The drawing under review shows one solid part. Ordinate dimensions are in mm from its lowest x, y, z. A direction names the side the tool comes from. Round coordinates to 2 decimals unless told otherwise and drop trailing zeros. Order: outer loops, then holes, each group sorted by start corner. A loop starts at its lowest first (then second) coordinate and runs counter-clockwise, first axis right, second up. Notation, with made-up numbers: M 78.5,35.25 L 123.5,35.25 A22 cw 123.5,45.25 Z; hole C 9,4.25 d1. An arc over 180 degrees is marked long. Use a Markdown table: item, result.
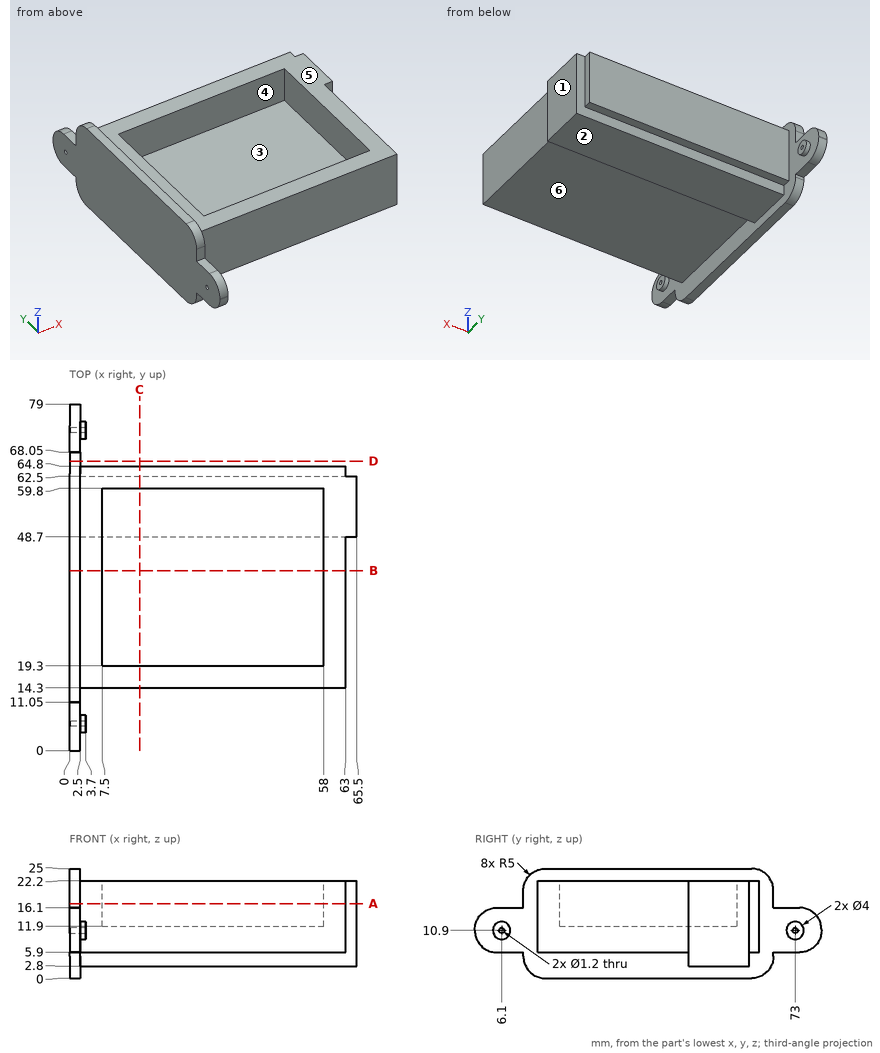
Q1. Draft analysis for pull direction X (two halves, no side actions). For the marked faces 1, 2 and 3, state which applies: pulls with the +X half, pulls with the -X half, needs draft (parallel to the pull), parting line crosses it, or undercut.
Determined:
| item | result |
|---|---|
| face 1 | pulls with the +X half |
| face 2 | needs draft |
| face 3 | undercut |
Q2. Add section D-D (y = 66). Write out the cut boundary in (x, z).
Determined:
| item | result |
|---|---|
| outline | M 0,0.96 L 2.5,0.96 L 2.5,24.04 L 0,24.04 Z |
Q3. Machinability: for the marked faces 4, 5 and 6, which of the approach directions +Z, -Z, +X, -X, +Y, -Y give a long, thin tool a straight path to every point of the face, cutting with its end or side? Answer none if there is none.
Determined:
| item | result |
|---|---|
| face 4 | +Z |
| face 5 | +Z, +X, +Y, -Y |
| face 6 | -Z, +X, -Y |
Q4. Add section A-A (z = 17). Write out the cut boundary in (x, y), then the cut area to 3 significant figures.
Determined:
| item | result |
|---|---|
| outline | M 0,11.05 L 2.5,11.05 L 2.5,14.3 L 63,14.3 L 63,48.7 L 65.5,48.7 L 65.5,62.5 L 63,62.5 L 63,64.8 L 2.5,64.8 L 2.5,68.05 L 0,68.05 Z; hole M 7.5,19.3 L 58,19.3 L 58,59.8 L 7.5,59.8 Z |
| area | 1,190 mm^2 |
Q5. Add section C-C (x = 16). Write out the cut boundary in (y, z), then the cut area to 3 significant figures.
Determined:
| item | result |
|---|---|
| outline | M 14.3,5.9 L 48.7,5.9 L 48.7,2.8 L 62.5,2.8 L 62.5,5.9 L 64.8,5.9 L 64.8,22.2 L 59.8,22.2 L 59.8,11.9 L 19.3,11.9 L 19.3,22.2 L 14.3,22.2 Z |
| area | 449 mm^2 |
Q6. Clearance check with flat-ended pins moving along their axes: pin 1 (1.2 mm diameter, centred on y = 73, z = 12, fed in from +X); pin 2 (3 mm diameter, centred on y = 39, z = 15.5, fed in from -X); pin 3 (2 mm diameter, centred on x = 0.5, y = 72, fed in from -Z); pin 4 (15 mm diameter, centred on x = 44, y = 31, fed in from +Z). State where each tip first meets the part, or that it passes through.
Determined:
| item | result |
|---|---|
| pin 1 | stops at x = 3.7 |
| pin 2 | stops at x = 0 |
| pin 3 | stops at z = 5.9 |
| pin 4 | stops at z = 11.9 |
Q7. Wall thickness on line 1 along Y through (x, z) = (2.15, 10.9); line 2 along X through (y, z) = (51, 20.5); line 3 along X through (y, z) = (43.5, 21.75): over which ranges is each line inside the solid? List them lowest first. Write a range as [from, to].
Determined:
| item | result |
|---|---|
| line 1 | y = [0, 5.5], [6.7, 72.4], [73.6, 79] |
| line 2 | x = [0, 7.5], [58, 65.5] |
| line 3 | x = [0, 7.5], [58, 63] |
Q8. Add section B-B (y = 41). Write out the cut boundary in (x, z), then the cut area to 4 significant figures.
Determined:
| item | result |
|---|---|
| outline | M 0,0 L 2.5,0 L 2.5,5.9 L 63,5.9 L 63,22.2 L 58,22.2 L 58,11.9 L 7.5,11.9 L 7.5,22.2 L 2.5,22.2 L 2.5,25 L 0,25 Z |
| area | 528.5 mm^2 |
